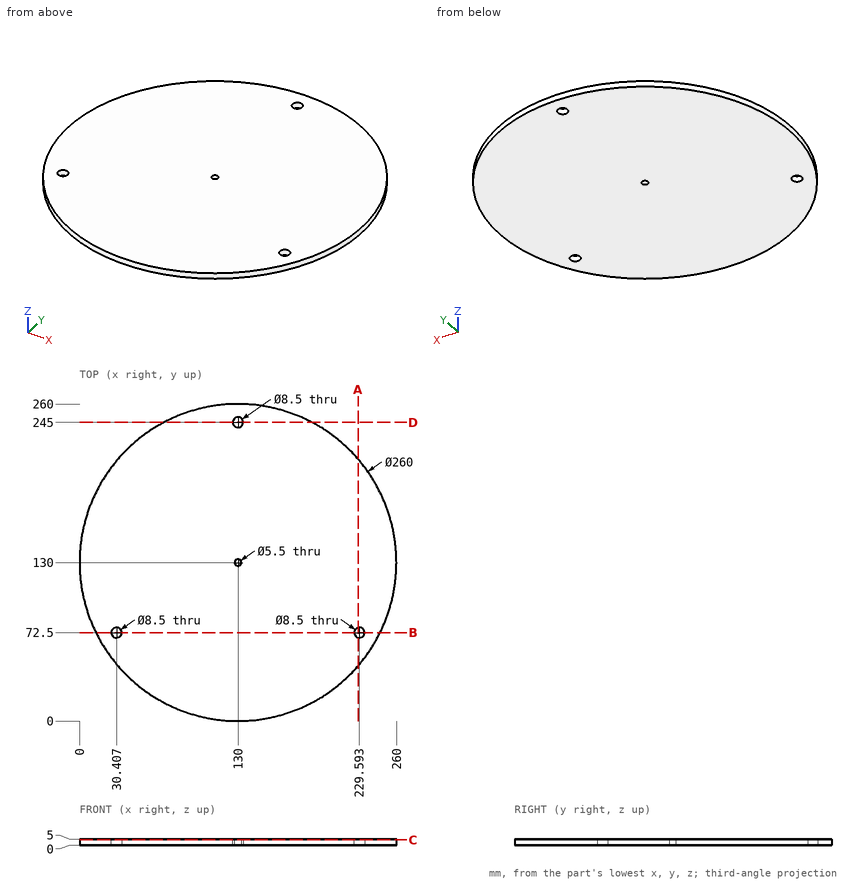
Drawing for the job (mm, zero at the part's lowest x, y, z). Give positions to 0.01 mm unless a question says otherwise; leave off trailing zeros. Loops run counter-clockwise (first coordinate to the right, second up) from the corner with the lowest first, then second, coordinate; pieces in that order, holes last.
Item 1: Drill centre lines: line 1 along Y through (x, z) = (130, 1.25); line 2 along Y through (x, z) = (216, 0.6); line 3 along Y through (x, z) = (226, 3.9). Where is each one in solid material? Low to high.
Check values:
line 1: y = 0 to 127.25, 132.75 to 240.75, 249.25 to 260
line 2: y = 32.51 to 227.49
line 3: y = 42.34 to 70.23, 74.77 to 217.66
Item 2: Slice it at A-A (x = 228.5). Write the cut outline in (y, z).
Check values:
outline: (45.16, 0) - (68.39, 0) - (68.39, 5) - (45.16, 5) - close; (76.61, 0) - (214.84, 0) - (214.84, 5) - (76.61, 5) - close
Item 3: Slice it at B-B (y = 72.5). Write the cut outline in (x, z).
Check values:
outline: (13.41, 0) - (26.16, 0) - (26.16, 5) - (13.41, 5) - close; (34.66, 0) - (225.34, 0) - (225.34, 5) - (34.66, 5) - close; (233.84, 0) - (246.59, 0) - (246.59, 5) - (233.84, 5) - close
Item 4: Slice it at D-D (y = 245). Write the cut outline in (x, z).
Check values:
outline: (69.38, 0) - (125.75, 0) - (125.75, 5) - (69.38, 5) - close; (134.25, 0) - (190.62, 0) - (190.62, 5) - (134.25, 5) - close
Item 5: Slice it at C-C (z = 4.2). Write the cut outline in (x, y), plus the area to 3 significant figures.
Check values:
outline: circle Ø260 at (130, 130); hole circle Ø8.5 at (30.41, 72.5); hole circle Ø8.5 at (130, 245); hole circle Ø5.5 at (130, 130); hole circle Ø8.5 at (229.59, 72.5)
area: 52,900 mm2
Item 6: Drop flat-ended pins along their axis: P1, Ø2, axis at x = 89, z = 1, coming from the +Y side; P2, Ø7, axis at x = 229.59, y = 72.5, coming from the +Z side; P3, Ø1.5, axis at y = 211, z = 1.5, coming from the -X side. Give the stop position or say it passes through.
Check values:
P1: stops at y = 253.69
P2: passes through
P3: stops at x = 27.73
